Input: part model. Units: mm. Frame: model coordinates. A direction names the side the tool comes from. Give positions to 0.01 mm unless a question says otherwise; leave off trailing zeros. Order: outer loops, then holes, each group sorted by start corner. A loop starts at its lowest first (then second) coordinate and runs counter-clockwise, first axis right, second up. Notation, with made-up numbers: (1, -6) -> (38, -6) arc R22 cw to (38, 30) -> close; hole circle Ø8 at (78.25, 81). An arc over 180 degrees is marked (long way). Use a Markdown table: item, result. Add a question column.
from build123d import *

# Parameters (mm, degrees)
F1_DEPTH = 5
F2_SIZE  = 2
F3_R     = 3
F4_R     = 2


with BuildPart() as f1:
    # F0 (on Top) → F1 (new body, symmetric)
    with BuildSketch(Plane.XY):
        with BuildLine():
            Line((10.4616216792, 7.1794074701), (0, 3.780220532))
            Line((0, 3.780220532), (-24.72135955, 79.8647418356))
            Line((-24.72135955, 79.8647418356), (-27.5745290989, 78.9376908525))
            Line((-27.5745290989, 78.9376908525), (-16.5475048962, 45))
            Line((-16.5475048962, 45), (-44.6666257322, 0))
            Line((-44.6666257322, 0), (-1.9261185658, 0))
            Line((-1.9261185658, 0), (15.0738814342, 0))
            ThreePointArc((15.0738814342, 0), (14.8645832244, 2.6593859057), (14.2418422113, 5.2532889044))
            Line((14.2418422113, 5.2532889044), (11.4606892619, 13.812797551))
            Line((11.4606892619, 13.812797551), (8.607519713, 12.8857465679))
            Line((8.607519713, 12.8857465679), (10.4616216792, 7.1794074701))
        make_face()
        Polygon((-6.0552643272, 3), (-39.2544824663, 3), (-17.4126071962, 37.9543071739), align=None, mode=Mode.SUBTRACT)
    extrude(amount=F1_DEPTH, both=True)

    # F2
    f2_edges = [f1.edges().sort_by_distance(p)[0] for p in [
        (10.034104, 13.349272, 5),
        (10.034104, 13.349272, -5),
        (-26.147944, 79.401216, 5),
        (-26.147944, 79.401216, -5),
    ]]
    chamfer(f2_edges, length=F2_SIZE)

    # F3
    f3_edges = [f1.edges().sort_by_distance(p)[0] for p in [
        (-17.412607, 37.954307, 0),
        (-39.254482, 3, 0),
        (-6.055264, 3, 0),
        (-44.666626, 0, 0),
        (-16.547505, 45, 0),
        (15.073881, 0, 0),
    ]]
    fillet(f3_edges, radius=F3_R)

    # F4
    f4_edges = [f1.edges().sort_by_distance(p)[0] for p in [
        (0, 3.780221, 0),
        (10.461622, 7.179407, 0),
    ]]
    fillet(f4_edges, radius=F4_R)


solid = f1.part
Q1. Section query D-D (y = 24.5). Return loops of the section in (x, z), plus the area to 3 significant figures.
Q2. Draft query along Y for faces 4 (the flat face through (10.054, 13.356, 0.042)), 5 (the cylindrical face through (-41.86, 1.51, 0.07)), 6 (the flat face through (-22.35, 62.86, 0.07)). Return one class per face: +Y half, -Y half, draft (parallel to the pull), parting line (faces both ways), or undercut.
Q3. Access query for faces 1 (the flat face through (10.367, 12.391, -4.014)), 2 (the cylindrical face through (-17.86, 33.88, -0.07)), 3 (the flat face through (10.367, 12.391, 4.014)). Directions: +Z, -Z, +X, -X, +Y, -Y. A direction counts if a zero-diameter tool reaches every point of the face in a straight line with its end or side. Return the directions, or none.
Q4. First-contact query: pin 1 (3 mm diameter, centred on x = -33, z = 1.5, fed in from -Y); pin 2 (4 mm diameter, centred on y = 68, z = 4, fed in from +X); pin 3 (6 mm diameter, centred on y = 50.5, z = -3, fed in from -X); pin 4 (1 mm diameter, centred on y = 68.5, z = -2.5, fed in from +X). Flat tips, straight axial feed; report the tip coordinate or a pass-through.
Q5. Section query A-A (z = -0.5). Return loops of the section in (x, y), plus the area to 3 significant figures.
Q6. Section query B-B (y = 10). Return loops of the section in (x, z), plus the area to 3 significant figures.
Q7. Section query C-C (x = -35). Return loops of the section in (y, z).
Q8. Ray query, line 1 (X direction, y = 9.5, z = 3.5); line 2 (Y direction, x = 1, z = -0.25); line 3 (Y direction, x = -28.5, z = 0.5). Return the intervals inside material, ascending.
Solution:
| question | item | result |
|---|---|---|
| 1 | outline | (-29.36, -5) -> (-25.82, -5) -> (-25.82, 5) -> (-29.36, 5) -> close; (-13.04, -5) -> (-6.73, -5) -> (-6.73, 5) -> (-13.04, 5) -> close |
| 1 | area | 98.5 mm² |
| 2 | face 4 | +Y half |
| 2 | face 5 | parting line |
| 2 | face 6 | undercut |
| 3 | face 1 | -Z, +Y |
| 3 | face 2 | +Z, -Z |
| 3 | face 3 | +Z, +Y |
| 4 | pin 1 | stops at y = 0 |
| 4 | pin 2 | stops at x = -20.22 |
| 4 | pin 3 | stops at x = -19.31 |
| 4 | pin 4 | stops at x = -20.87 |
| 5 | outline | (-41.8, 4.59) arc R3 ccw to (-39.25, 0) -> (11.75, 0) arc R3 ccw to (14.68, 3.64) arc R17 ccw to (14.24, 5.25) -> (11.46, 13.81) -> (8.61, 12.89) -> (9.84, 9.08) arc R2 cw to (8.56, 6.56) -> (1.9, 4.4) arc R2 cw to (-0.62, 5.68) -> (-24.72, 79.86) -> (-27.57, 78.94) -> (-16.98, 46.33) arc R3 cw to (-17.29, 43.81) -> close; hole (-36.39, 7.59) arc R3 ccw to (-33.84, 3) -> (-10.18, 3) arc R3 ccw to (-7.33, 6.93) -> (-15.42, 31.84) arc R3 ccw to (-20.82, 32.5) -> close |
| 5 | area | 748 mm² |
| 6 | outline | (-38.42, -5) -> (-34.88, -5) -> (-34.88, 5) -> (-38.42, 5) -> close; (-8.33, -5) -> (-2.02, -5) -> (-2.02, 5) -> (-8.33, 5) -> close; (9.55, -5) -> (12.7, -5) -> (12.7, 5) -> (9.55, 5) -> close |
| 6 | area | 130 mm² |
| 7 | outline | (0, -5) -> (3.23, -5) -> (3.23, 5) -> (0, 5) -> close; (9.81, -5) -> (15.47, -5) -> (15.47, 5) -> (9.81, 5) -> close |
| 8 | line 1 | x = -38.73 to -35.19, -8.17 to -1.86, 9.71 to 12.86 |
| 8 | line 2 | y = 0 to 4.32 |
| 8 | line 3 | y = 0 to 3, 20.21 to 25.87 |
